Can you work these out from the model? Positions are in its coordinate system, mm. Give positions to 0.01 mm unless a question says otherwise; leave off trailing zeros. Loops run counter-clockwise (first coordinate to the right, second up) from the corner with the lowest first, then second, coordinate; pieces in that order, holes last.
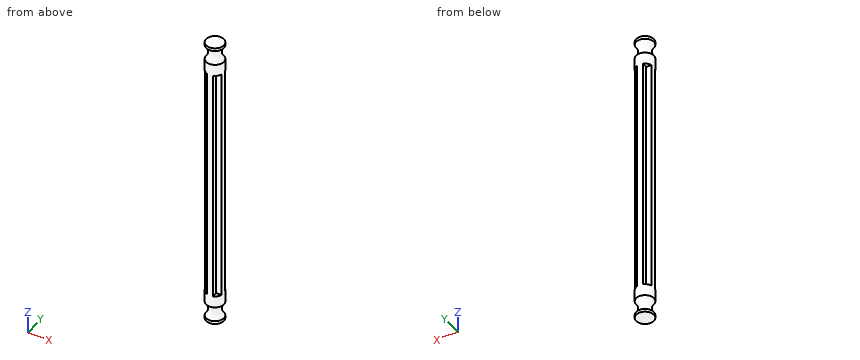
from build123d import *

# Parameters (mm, degrees)
F2_W          = 2
F2_H          = 2
F3_DEPTH      = 40
F3_DEPTH_BACK = 40


# Not quite as in the source:
# - a feature names something its author has since deleted; it is built from what else it names


with BuildPart() as f1:
    # F0 (on Front) → F1 (revolve)
    with BuildSketch(Plane.XZ):
        with BuildLine():
            Line((0, 50), (0, -50))
            Line((0, -50), (3, -50))
            Line((3, -50), (3, -49))
            ThreePointArc((3, -49), (2, -46.5), (3, -44))
            Line((3, -44), (3, 0))
            Line((3, 0), (3, 44))
            ThreePointArc((3, 44), (2, 46.5), (3, 49))
            Line((3, 49), (3, 50))
            Line((3, 50), (0, 50))
        make_face()
    revolve(axis=Axis((0, 0, 0), (0, 0, 1)))

    # F2 (on Top) → F3 (cut, two sides)
    with BuildSketch(Plane.XY) as f3_sk:
        with Locations((2, 2)):
            Rectangle(F2_W, F2_H)
        with Locations((-2, 2)):
            Rectangle(F2_W, F2_H)
        with Locations((-2, -2)):
            Rectangle(F2_W, F2_H)
        with Locations((2, -2)):
            Rectangle(F2_W, F2_H)
    extrude(amount=-F3_DEPTH, mode=Mode.SUBTRACT)
    extrude(f3_sk.sketch, amount=F3_DEPTH_BACK, mode=Mode.SUBTRACT)


solid = f1.part
(1) Will these pins go through, and if not, where does the flat tip stop? P1, Ø0.9, axis at y = 2, z = -13.5, coming from the -X side; P2, Ø0.5, axis at x = 2.5, z = -17.5, coming from the -Y side; P3, Ø0.5, axis at x = 2.5, z = 20, coming from the +Y side.
Returned:
P1: stops at x = -1
P2: stops at y = -1
P3: stops at y = 1
(2) Please list where these lines run through material, in increasing order: probe 1 along Z at (x, y) = (1.95, -1.6); probe 2 along Z at (x, y) = (-2.4, 1.2); probe 3 along X at (y, z) = (-1.65, -25).
Returned:
probe 1: z = -50 to -48.37, -44.63 to -40, 40 to 44.63, 48.37 to 50
probe 2: z = -50 to -48.62, -44.38 to -40, 40 to 44.38, 48.62 to 50
probe 3: x = -1 to 1
(3) Suppose I cut it at A-A on y = 0. List the corners of the cut face in (x, z) for me (3 decimals), plus the area to 3 significant figures.
Returned:
outline: (-3, -50) - (3, -50) - (3, -49) arc R3.625 cw to (3, -44) - (3, 44) arc R3.625 cw to (3, 49) - (3, 50) - (-3, 50) - (-3, 49) arc R3.625 cw to (-3, 44) - (-3, -44) arc R3.625 cw to (-3, -49) - close
area: 586 mm2
